For this review, take the finished solid that the model builds, in its own axes (mm). Face numbers are marked on the shaded views. A direction names the side the tool comes from. Give positions to 0.01 mm unless a question says otherwise; leave off trailing zeros. Loops run counter-clockwise (first coordinate to the right, second up) from the corner with the lowest first, then second, coordinate; pieces in that order, holes last. Notation, with made-up numbers: (27.5, 75.25) - (43.5, 75.25) arc R15 cw to (43.5, 93.25) - close; hole circle Ø3 at (-39, 70.25). An arc over 180 degrees is marked (long way). Use CSV: the item, a comma, the result in double quotes. Start each with the question number.
1. For the marked faces 3 and 4, list the 3-axis set-ups (+Z, -Z, +X, -X, +Y, -Y) from which the entire face can be reached by the end or side of a thin tool; tool diameter is ignored.
2. Take a section at C-C on y = 5. Give the boundary of the cut face in (x, z).
3. Wall thickness on line 1 (Y direction, x = 0, z = -76); line 2 (Z direction, x = -29, y = -24); line 3 (Y direction, x = 17.5, z = 56): over which ranges is each line inside the solid? List them lowest first.
4. Mouldability with a two-part tool opening along Y and no side actions: class the marked faces 1 and 2 as pulls with the +Y half, pulls with the -Y half, needs draft (parallel to the pull), parting line crosses it, or undercut.
5. Take a section at B-B on y = 59.5. Give the boundary of the cut face in (x, z), plus the area to 3 significant figures.
6. Take a section at D-D on z = 66.5. Give the boundary of the cut face in (x, y).
7. For pin 1 (5 mm diameter, centred on x = 12, z = 21.5, fed in from -Y); pin 2 (6 mm diameter, centred on y = 251, z = 28, fed in from -X); pin 3 (12 mm diameter, centred on x = -4.5, z = -51, fed in from -Y), all flat-tipped, find the tip position at first contact; note any pin that passes through.
8. Take a section at A-A on x = 0. Give the boundary of the cut face in (y, z).
```python
from build123d import *

# Parameters (mm, degrees)
BOSS_EXTRUDE1_START = 75
SKETCH1_R           = 20
BOSS_EXTRUDE1_DEPTH = 5
SKETCH2_R           = 20
BOSS_EXTRUDE2_DEPTH = 140


with BuildPart() as part:
    # Sketch1 → Boss-Extrude1 (new body, symmetric)
    with BuildSketch(Plane.XY.offset(BOSS_EXTRUDE1_START)):
        with BuildLine():
            Line((-40, 0), (-40, 250))
            ThreePointArc((-40, 250), (0, 290), (40, 250))
            Line((40, 250), (40, 0))
            ThreePointArc((40, 0), (0, -40), (-40, 0))
        make_face()
        Circle(SKETCH1_R, mode=Mode.SUBTRACT)
    boss_extrude1 = extrude(amount=BOSS_EXTRUDE1_DEPTH, both=True)

    # Sketch2 → Boss-Extrude2 (add)
    with BuildSketch(Plane(origin=(0, 0, 70), x_dir=(-1, 0, 0), z_dir=(0, 0, -1))):
        with Locations((0, 250)):
            Circle(SKETCH2_R)
        with Locations((0, 150)):
            Circle(SKETCH2_R)
    extrude(amount=BOSS_EXTRUDE2_DEPTH)

    # Mirror2: Boss-Extrude1 across plane
    add(boss_extrude1.mirror(Plane.XY))


solid = part.part
```
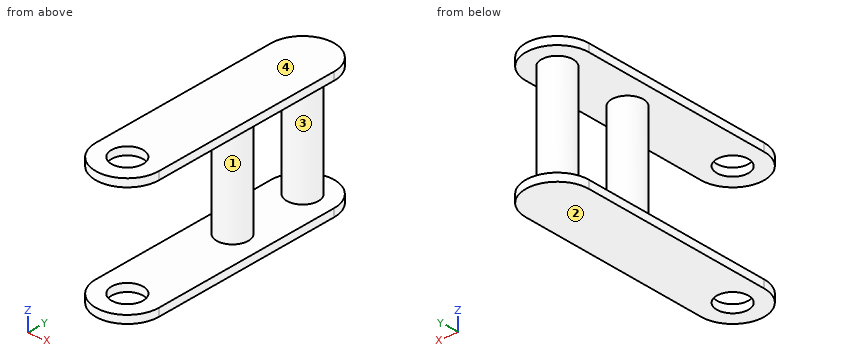
Check result:
1,face 3,"none"
1,face 4,"+Z, +X, -X, +Y, -Y"
2,outline,"(-40, -80) - (-19.36, -80) - (-19.36, -70) - (-40, -70) - close; (-40, 70) - (-19.36, 70) - (-19.36, 80) - (-40, 80) - close; (19.36, -80) - (40, -80) - (40, -70) - (19.36, -70) - close; (19.36, 70) - (40, 70) - (40, 80) - (19.36, 80) - close"
3,line 1,"y = -40 to -20, 20 to 290"
3,line 2,"z = -80 to -70, 70 to 80"
3,line 3,"y = 140.32 to 159.68, 240.32 to 259.68"
4,face 1,"undercut"
4,face 2,"needs draft"
5,outline,"(-40, -80) - (40, -80) - (40, -70) - (-40, -70) - close; (-40, 70) - (40, 70) - (40, 80) - (-40, 80) - close"
5,area,"1,600 mm²"
6,outline,"circle Ø40 at (0, 150); circle Ø40 at (0, 250)"
7,pin 1,"stops at y = 132.4"
7,pin 2,"stops at x = -20"
7,pin 3,"stops at y = 130"
8,outline,"(-40, -80) - (-20, -80) - (-20, -70) - (-40, -70) - close; (-40, 70) - (-20, 70) - (-20, 80) - (-40, 80) - close; (20, -80) - (290, -80) - (290, -70) - (270, -70) - (270, 70) - (290, 70) - (290, 80) - (20, 80) - (20, 70) - (130, 70) - (130, -70) - (20, -70) - close; hole (170, -70) - (230, -70) - (230, 70) - (170, 70) - close"
